Geometry check sheet. Reference: drawing and pictorial views, mm from the part's lowest x, y, z. Round coordinates to 2 decimals unless told otherwise and drop trailing zeros. Order: outer loops, then holes, each group sorted by start corner. A loop starts at its lowest first (then second) coordinate and runs counter-clockwise, first axis right, second up.
(1) Sectioned sample at A-A, the plane z = 7.5. Enter the section's corners in (x, y), and give its area (3 significant figures).
(2) Mould release check, pull along X, two halves, no side actions. Record for the marked faces 1, 2 and 3: released by +X, released by -X, zero draft, split by the parting line, or undercut.
(3) Sectioned sample at C-C, the plane y = 1.25. Enter the section's corners in (x, z).
(4) Sectioned sample at D-D, the plane z = 14.25. Enter the section's corners in (x, y), and give its area (3 significant figures).
(5) Sectioned sample at B-B, the plane x = 45. Enter the section's corners in (y, z), and give its area (3 significant figures).
(6) Depth check by flat-ended pin: pin 1 (3.5 mm diameter, centred on x = 5, z = 7.5, fed in from -Y); pin 2 (3 mm diameter, centred on x = 45, z = 7.5, fed in from +Y). Enter the tip coordinate at first touch or a pass-through.
(7) Thickness scan on probe 1 along X at (y, z) = (1.4, 7.5); probe 2 along X at (y, z) = (1.35, 8.5); probe 3 along Z at (x, y) = (25.5, 1.1). Record the ranges inside material, lowest first.
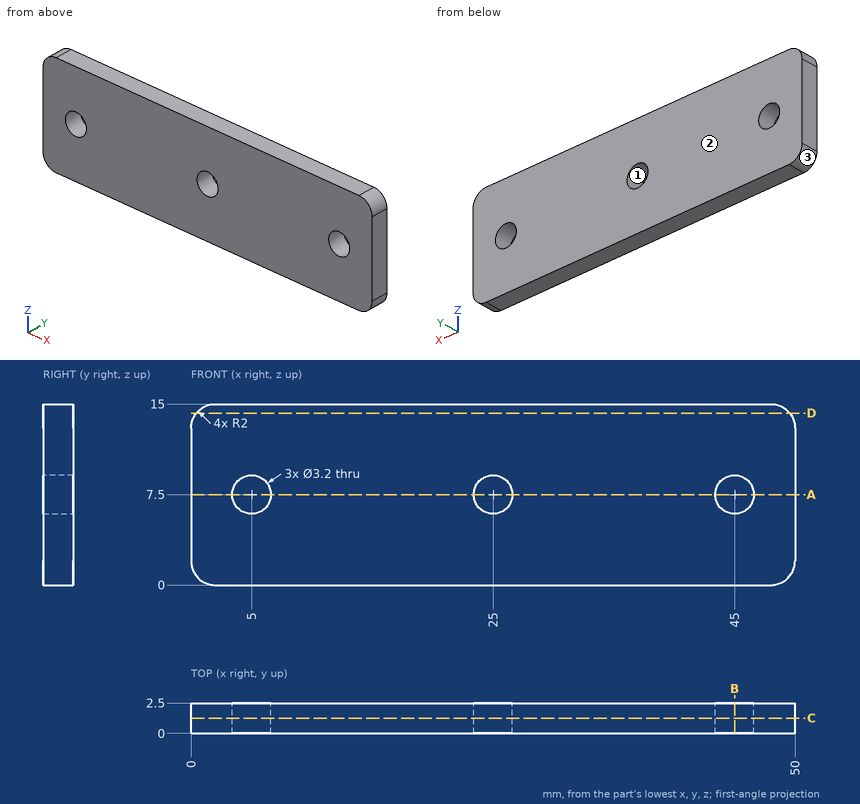
Derived:
1. outline: (0, 0) - (3.4, 0) - (3.4, 2.5) - (0, 2.5) - close; (6.6, 0) - (23.4, 0) - (23.4, 2.5) - (6.6, 2.5) - close; (26.6, 0) - (43.4, 0) - (43.4, 2.5) - (26.6, 2.5) - close; (46.6, 0) - (50, 0) - (50, 2.5) - (46.6, 2.5) - close
1. area: 101 mm2
2. face 1: undercut
2. face 2: zero draft
2. face 3: released by -X
3. outline: (0, 2) arc R2 ccw to (2, 0) - (48, 0) arc R2 ccw to (50, 2) - (50, 13) arc R2 ccw to (48, 15) - (2, 15) arc R2 ccw to (0, 13) - close; hole circle Ø3.2 at (5, 7.5); hole circle Ø3.2 at (25, 7.5); hole circle Ø3.2 at (45, 7.5)
4. outline: (0.44, 0) - (49.56, 0) - (49.56, 2.5) - (0.44, 2.5) - close
4. area: 123 mm2
5. outline: (0, 0) - (2.5, 0) - (2.5, 5.9) - (0, 5.9) - close; (0, 9.1) - (2.5, 9.1) - (2.5, 15) - (0, 15) - close
5. area: 29.5 mm2
6. pin 1: stops at y = 0
6. pin 2: passes through
7. probe 1: x = 0 to 3.4, 6.6 to 23.4, 26.6 to 43.4, 46.6 to 50
7. probe 2: x = 0 to 3.75, 6.25 to 23.75, 26.25 to 43.75, 46.25 to 50
7. probe 3: z = 0 to 5.98, 9.02 to 15
